```python
from build123d import *


with BuildPart() as part:
    # Esquisse1 → Révolution1 (revolve)
    with BuildSketch(Plane.XY, mode=Mode.PRIVATE) as r_volution1_sk:
        with BuildLine():
            Line((0, 6), (22.5, 6))
            Line((22.5, 6), (22.5, 15))
            Line((22.5, 15), (21.5, 15))
            ThreePointArc((21.5, 15), (21.146446609, 14.853553391), (21, 14.5))
            Line((21, 14.5), (21, 13))
            Line((21, 13), (1, 13))
            Line((1, 13), (0, 12))
            Line((0, 12), (0, 6))
        make_face()
    revolve(r_volution1_sk.sketch.rotate(Axis((0, 0, 0), (1, 0, 0)), 90), axis=Axis((0, 0, 0), (1, 0, 0)))  # turned: the seam where the file's is


solid = part.part
```
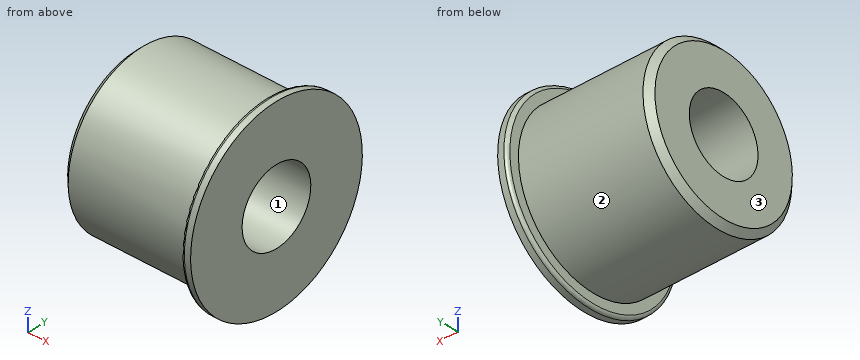
Source: CAD feature listing. Evaluate the final solid. Frame: model axes, mm. Face numbers are marked on the shaded views. Give positions to 0.01 mm unless a question says otherwise; leave off trailing zeros. Order: outer loops, then holes, each group sorted by start corner. A loop starts at its lowest first (then second) coordinate and runs counter-clockwise, first axis right, second up.
(1) Pull-direction query (Z, two-part tool) for the marked faces 1, 2 and 3; classes: +Z half, -Z half, draft (parallel to the pull), parting line (faces both ways), or undercut.
(2) Contact query for flat-ended pins moving along their axis: P1, Ø8, axis at x = 16, y = -8, coming from the +Z side; P2, Ø1.5, axis at x = 15, y = 2.5, coming from the +Z side; P3, Ø1.5, axis at x = 18, y = 4, coming from the +Z side. Output: stop coordinate, or through.
(3) Section query C-C (x = 6.5). Return the cut outline in (y, z), plus the area to 3 significant figures.
(4) Section query A-A (y = 0). Return the cut outline in (x, z).
(5) Material intervals for line 1 along Y through (x, z) = (12, 0); line 2 along X through (y, z) = (-8.5, -10.5); line 3 along Z through (x, y) = (13.5, 1.5), sorted ascending.
Outcome:
1. face 1: undercut
1. face 2: parting line
1. face 3: draft
2. P1: stops at z = 12.37
2. P2: stops at z = 12.88
2. P3: stops at z = 12.59
3. outline: circle Ø26 at (0, 0); hole circle Ø12 at (0, 0)
3. area: 418 mm2
4. outline: (0, -12) - (1, -13) - (21, -13) - (21, -14.5) arc R0.5 ccw to (21.5, -15) - (22.5, -15) - (22.5, -6) - (0, -6) - close; (0, 6) - (22.5, 6) - (22.5, 15) - (21.5, 15) arc R0.5 ccw to (21, 14.5) - (21, 13) - (1, 13) - (0, 12) - close
5. line 1: y = -13 to -6, 6 to 13
5. line 2: x = 21 to 22.5
5. line 3: z = -12.91 to -5.81, 5.81 to 12.91
